The listing builds one solid part. Answer for the finished solid, in the listing's coordinates (mm). A direction names the side the tool comes from. Coordinates: 2 decimals unless noted, no trailing zeros. Order: outer loops, then holes, each group sorted by start corner. A loop starts at its lowest first (then second) coordinate and runs counter-clockwise, first axis right, second up. Notation, with made-up numbers: (-12.5, 1) -> (11.5, 1) arc R34 cw to (11.5, 36) -> close; hole circle Ø11 at (-13, 37.25). An arc over 180 degrees is marked (long way). Return JSON: item names as keys, results as strings.
```python
from build123d import *

# Parameters (mm, degrees)
ESQUISSE1_W        = 20
ESQUISSE1_H        = 150
BOSS_EXTRU_1_DEPTH = 5
ESQUISSE2_W        = 20
ESQUISSE2_H        = 150
BOSS_EXTRU_2_DEPTH = 5


with BuildPart() as part:
    # Esquisse1 → Boss.-Extru.1 (new body)
    with BuildSketch(Plane.XY):
        with Locations((-41.945195284, -26.747319263)):
            Rectangle(ESQUISSE1_W, ESQUISSE1_H)
        with BuildLine():
            Line((-45.495195284, 38.252680737), (-44.945195284, 22.252680737))
            ThreePointArc((-44.945195284, 22.252680737), (-41.945195284, 19.252680737), (-38.945195284, 22.252680737))
            Line((-38.945195284, 22.252680737), (-38.395195284, 38.252680737))
            ThreePointArc((-38.395195284, 38.252680737), (-41.945195284, 41.802680737), (-45.495195284, 38.252680737))
        make_face(mode=Mode.SUBTRACT)
    extrude(amount=BOSS_EXTRU_1_DEPTH)

    # Esquisse2 → Boss.-Extru.2 (add)
    with BuildSketch(Plane.XY.offset(5)):
        with Locations((-41.945195284, -26.747319263)):
            Rectangle(ESQUISSE2_W, ESQUISSE2_H)
    extrude(amount=BOSS_EXTRU_2_DEPTH)


solid = part.part
```
Item 1: The part is cut by section A-A on z = 3. Determine the outline of the cut face in (x, y).
Answer list:
{"outline": "(-51.95, -101.75) -> (-31.95, -101.75) -> (-31.95, 48.25) -> (-51.95, 48.25) -> close; hole (-45.5, 38.25) -> (-44.95, 22.25) arc R3 ccw to (-38.95, 22.25) -> (-38.4, 38.25) arc R3.55 ccw to start"}
Item 2: Find the intervals of material crossed by probe 1 along Y at (x, z) = (-42.5, 1.5), in increasing order.
Answer list:
{"probe 1": "-101.75 to 19.3, 41.76 to 48.25"}
Item 3: Which of the six approach directions +Z, -Z, +X, -X, +Y, -Y give full straight-line access (tool end or side, diameter ignored) to faces 1 (the flat face through (-42, 31, 5)), 2 (the flat face through (-42, -26, 10))?
Answer list:
{"face 1": "-Z", "face 2": "+Z, +X, -X, +Y, -Y"}
Item 4: Determine the mould class of faces 3 (the flat face through (-42, -101.747, 5)), 4 (the cylindrical face through (-41.87, 41.8, 2.46)), 5 (the flat face through (-31.945, -28, 5)) for opening direction X: pulls with the +X half, pulls with the -X half, needs draft (parallel to the pull), parting line crosses it, or undercut.
Answer list:
{"face 3": "needs draft", "face 4": "undercut", "face 5": "pulls with the +X half"}
Item 5: A flat-ended cylindrical pin translates along its axis: pin 1 (5.5 mm diameter, centred on x = -42.5, y = 32.5, fed in from -Z). Find the tip coordinate at first contact, or state that the pin passes through.
Answer list:
{"pin 1": "z = 5"}
